Print and shaded views of the part. All mm, measured from the part's lowest x, y and z. Round coordinates to 2 decimals unless told otherwise and drop trailing zeros. Loops run counter-clockwise (first coordinate to the right, second up) from the corner with the lowest first, then second, coordinate; pieces in that order, holes last. Notation, with made-up numbers: (71, -25) -> (101, -25) arc R10 ccw to (101, -20) -> close; hole circle Ø4 at (37, 66.5). An arc over 180 degrees is marked (long way). Use a Markdown table: item, result.
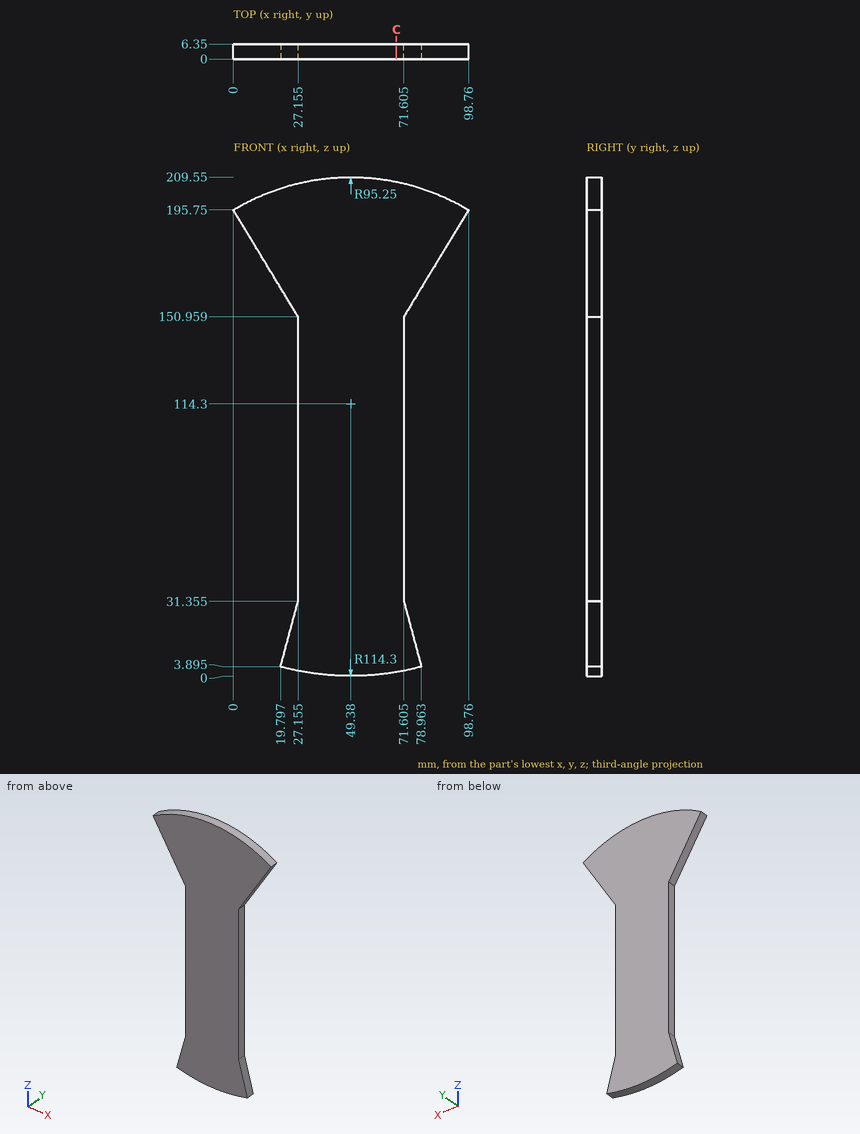
Q1. Drill centre lines: L1, parallel to X at y = 1.5, z = 99.5 (1 decimal); L2, parallel to Z at x = 34.5, y = 4.75; L3, parallel to Z at x = 47.5, y = 3 (1 decimal). Where is each one in solid material? Low to high. Write a range as from..to.
Results list:
| item | result |
|---|---|
| L1 | x = 27.2..71.6 |
| L2 | z = 0.97..208.38 |
| L3 | z = 0..209.5 |
Q2. Band-saw the part on C-C, the plane x = 68.5. Give the cut face in (y, z), plus the area to 3 significant figures.
Results list:
| item | result |
|---|---|
| outline | (0, 1.61) -> (6.35, 1.61) -> (6.35, 207.61) -> (0, 207.61) -> close |
| area | 1,310 mm² |
Q3. Flat gauge pins, fed straight in: pin 1 (1.5 mm diameter, centred on y = 1.5, z = 70, fed in from -X) (1 decimal); pin 2 (1.5 mm diameter, centred on x = 14.5, y = 1, fed in from -Z) (1 decimal). Where does each tip first touch, or does it go through?
Results list:
| item | result |
|---|---|
| pin 1 | stops at x = 27.2 |
| pin 2 | stops at z = 170.6 |
